from build123d import *

# Parameters (mm, degrees)
SKETCH1_W               = 16
SKETCH1_H               = 79
BOSS_EXTRUDE1_DEPTH     = 12
CUT_EXTRUDE1_DEPTH      = 81.305666052
CUT_EXTRUDE1_DEPTH_BACK = 81.305666052
CUT_EXTRUDE2_DEPTH      = 81.305666052
CUT_EXTRUDE2_DEPTH_BACK = 81.305666052
SKETCH4_R               = 3
SKETCH4_R_2             = 1.5
BOSS_EXTRUDE2_DEPTH     = 2.5
FILLET1_R               = 1
FILLET2_R               = 10
SKETCH5_W               = 5
SKETCH5_H               = 10
CUT_EXTRUDE3_DEPTH      = 5
CUT_EXTRUDE4_REACH      = 55.096
SKETCH6_W               = 5
SKETCH6_H               = 2.5
SKETCH7_W               = 5
SKETCH7_H               = 10
CUT_EXTRUDE5_DEPTH      = 81.305666052


with BuildPart() as part:
    # Sketch1 → Boss-Extrude1 (new body)
    with BuildSketch(Plane.XY):
        with Locations((0, -39.5)):
            Rectangle(SKETCH1_W, SKETCH1_H)
    extrude(amount=BOSS_EXTRUDE1_DEPTH)

    # Sketch2 → Cut-Extrude1 (cut, two sides: drawn at the far end of the back side and taken through both)
    with BuildSketch(Plane(origin=(0, 0, 0), x_dir=(0, 0, -1), z_dir=(1, 0, 0)).offset(-CUT_EXTRUDE1_DEPTH_BACK)):
        Polygon((-8, 0), (0, 0), (0, -8), align=None)
    extrude(amount=CUT_EXTRUDE1_DEPTH + CUT_EXTRUDE1_DEPTH_BACK, mode=Mode.SUBTRACT)

    # Sketch3 → Cut-Extrude2 (cut, two sides: drawn at the far end of the back side and taken through both)
    with BuildSketch(Plane(origin=(0, 0, 0), x_dir=(0, 0, -1), z_dir=(1, 0, 0)).offset(-CUT_EXTRUDE2_DEPTH_BACK)):
        with BuildLine():
            ThreePointArc((-3, 1.1), (-6.559834153, 4.04730143), (-8.791057147, 0))
            Line((-8.791057147, 0), (-7.019803903, 0))
            ThreePointArc((-7.019803903, 0), (-6.600122548, 2.474719218), (-4.5, 1.1))
            ThreePointArc((-4.5, 1.1), (-4.625280782, 0.499877452), (-4.980196097, 0))
            Line((-4.980196097, 0), (-3.208942853, 0))
            ThreePointArc((-3.208942853, 0), (-3.05269857, 0.540165847), (-3, 1.1))
        make_face()
        with BuildLine():
            Line((-7.019803903, 0), (-8.791057147, 0))
            ThreePointArc((-8.791057147, 0), (-6, -1.9), (-3.208942853, 0))
            Line((-3.208942853, 0), (-4.980196097, 0))
            ThreePointArc((-4.980196097, 0), (-6, -0.4), (-7.019803903, 0))
        make_face()
    extrude(amount=CUT_EXTRUDE2_DEPTH + CUT_EXTRUDE2_DEPTH_BACK, mode=Mode.SUBTRACT)

    # Sketch4 → Boss-Extrude2 (add, symmetric)
    with BuildSketch(Plane(origin=(0, 0, 0), x_dir=(0, 0, -1), z_dir=(1, 0, 0))):
        with Locations((-6, 1.1)):
            Circle(SKETCH4_R)
        with Locations((-6, 1.1)):
            Circle(SKETCH4_R_2, mode=Mode.SUBTRACT)
    extrude(amount=BOSS_EXTRUDE2_DEPTH, both=True)

    # Fillet1
    fillet1_edges = [part.edges().sort_by_distance(p)[0] for p in [
        (0, -1.898274836, 6.101725164),
        (0, 0, 8.791057147),
    ]]
    fillet(fillet1_edges, radius=FILLET1_R)

    # Fillet2
    fillet2_edges = [part.edges().sort_by_distance(p)[0] for p in [
        (0, -8, 0),
    ]]
    fillet(fillet2_edges, radius=FILLET2_R)

    # Sketch5 → Cut-Extrude3 (cut)
    with BuildSketch(Plane(origin=(0, 0, 0), x_dir=(-1, 0, 0), z_dir=(0, 0, -1))):
        with Locations((0, -32)):
            Rectangle(SKETCH5_W, SKETCH5_H)
        with Locations((0, -52)):
            Rectangle(SKETCH5_W, SKETCH5_H)
    extrude(amount=-CUT_EXTRUDE3_DEPTH, mode=Mode.SUBTRACT)

    # Sketch6 → Cut-Extrude4 (cut, up to next)
    with BuildSketch(Plane.XZ.offset(47), mode=Mode.PRIVATE) as cut_extrude4_sk1:
        with Locations((0, 3.75)):
            Rectangle(SKETCH6_W, SKETCH6_H)
    cut_extrude4_tool1 = extrude(cut_extrude4_sk1.sketch, amount=-CUT_EXTRUDE4_REACH, mode=Mode.PRIVATE) & part.part
    add(cut_extrude4_tool1.solids().sort_by_distance((0, -47, 3.75))[0], mode=Mode.SUBTRACT)

    # Sketch7 → Cut-Extrude5 (cut, through all)
    with BuildSketch(Plane(origin=(0, 0, 0), x_dir=(-1, 0, 0), z_dir=(0, 0, -1))):
        with Locations((0, -52)):
            Rectangle(SKETCH7_W, SKETCH7_H)
    extrude(amount=-CUT_EXTRUDE5_DEPTH, mode=Mode.SUBTRACT)


solid = part.part
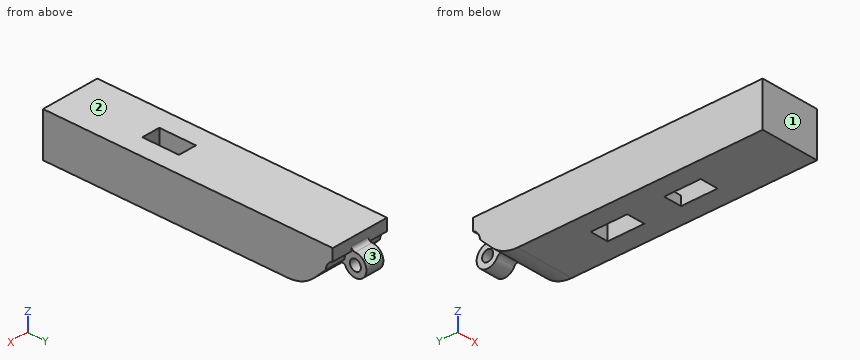
Read the model definition and answer for the solid it produces. Units are mm, in the model's axes. Face numbers are marked on the shaded views. Give positions to 0.01 mm unless a question says otherwise; leave off trailing zeros. Write each loop counter-clockwise with the first axis right and the second up, starting at its lowest first coordinate (ties: lowest second). Pieces come first, ordered by that corner, then holes. Notation, with made-up numbers: M -33,42 L 24,42 A28 cw 24,80 Z; hole C -4.5,-12.5 d3. An arc over 180 degrees is marked long. One line per item, written item: value. Start each with the question number.
(1) Flat-ended cylindrical pins translate along their axes: pin 1 Ø2.5 at (x, z) = (1, 7.5) entering from +Y; pin 2 Ø1.2 at (x, z) = (0, 1) entering from +Y; pin 3 Ø4 at (y, z) = (1.1, 6) entering from -X. Find the tip coordinate at first contact, or state that the pin passes through.
(2) Find section C-C (z = 10.75). Determine the outline of the cut face in (x, y).
(3) Determine the mould class of the marked faces 1, 2 and 3 for opening direction Y: pulls with the +Y half, pulls with the -Y half, needs draft (parallel to the pull), parting line crosses it, or undercut.
(4) Find section A-A (y = -55.5). Determine the outline of the cut face in (x, z).
(5) Find section B-B (x = -4). Determine the outline of the cut face in (y, z).
(6) Find the intervals of material crossed by line 1 (Y direction, x = -0.15, z = 6); line 2 (X direction, y = -50.5, z = 3.5); line 3 (Y direction, x = -0.75, z = 10), in increasing order.
Results below:
1. pin 1: stops at y = 4.09
1. pin 2: stops at y = -6.72
1. pin 3: stops at x = -2.5
2. outline: M -8,-79 L 8,-79 L 8,0 L -8,0 Z; hole M -2.5,-57 L 2.5,-57 L 2.5,-47 L -2.5,-47 Z
3. face 1: pulls with the -Y half
3. face 2: needs draft
3. face 3: undercut
4. outline: M -8,0 L -2.5,0 L -2.5,12 L -8,12 Z; M 2.5,0 L 8,0 L 8,12 L 2.5,12 Z
5. outline: M -79,0 L -12.14,0 A10 ccw -5.07,2.93 L -1.9,6.1 A3 cw 0,8.79 L 0,12 L -79,12 Z
6. line 1: y = -79 to -57, -47 to -0.4, 2.6 to 4.1
6. line 2: x = -8 to -2.5, 2.5 to 8
6. line 3: y = -79 to -57, -47 to 0
